The figure shows three views and two pictorial views of one solid part (mm, origin at its lowest corner). Answer the questions. Coordinates: 2 decimals unless noted, no trailing zeros. Loops run counter-clockwise (first coordinate to the right, second up) from the corner with the lowest first, then second, coordinate; pieces in that order, holes last. Notation, with made-up numbers: (55.25, 58) -> (81.25, 58) arc R14 ccw to (81.25, 71) -> close; hole circle Ø8 at (30, 28). An arc over 180 degrees is marked (long way). Answer as a JSON object with one key per item and string values. Group by question number.
1) Section B-B, the plane y = 1.5 is taken. Give the vertices of the cut face in (x, z), plus the area to 3 significant figures.
2) Determine the mould class of the marked faces 1 and 2 for opening direction Z: released by +Z, released by -Z, zero draft, split by the parting line, or undercut.
3) Flat-ended cylindrical pins translate along their axes: P1, Ø6, axis at x = 64.5, y = 3, coming from the +Z side; P2, Ø5, axis at y = 3, z = 43.5, coming from the +X side; P3, Ø1.5, axis at y = 3.5, z = 138.5, coming from the -X side; P4, Ø2, axis at y = 6.5, z = 99, coming from the +X side. Find the tip coordinate at first contact, or state that the pin passes through.
4) Section C-C, the plane x = 118 is taken. Give the vertices of the cut face in (y, z), plus the area to 3 significant figures.
5) Consider probe 1 along Z at (x, y) = (99, 9) (3 decimals); probe 2 along Z at (x, y) = (123, 3.25); probe 3 along Z at (x, y) = (97.5, 1.25). Determine where each line is inside the solid, lowest interval first. Write a range as [from, to].
6) Section A-A, the plane z = 160 is taken. Give the vertices of the cut face in (x, y).
7) Section D-D, the plane z = 100 is taken. Give the vertices of the cut face in (x, y), plus the area to 3 significant figures.
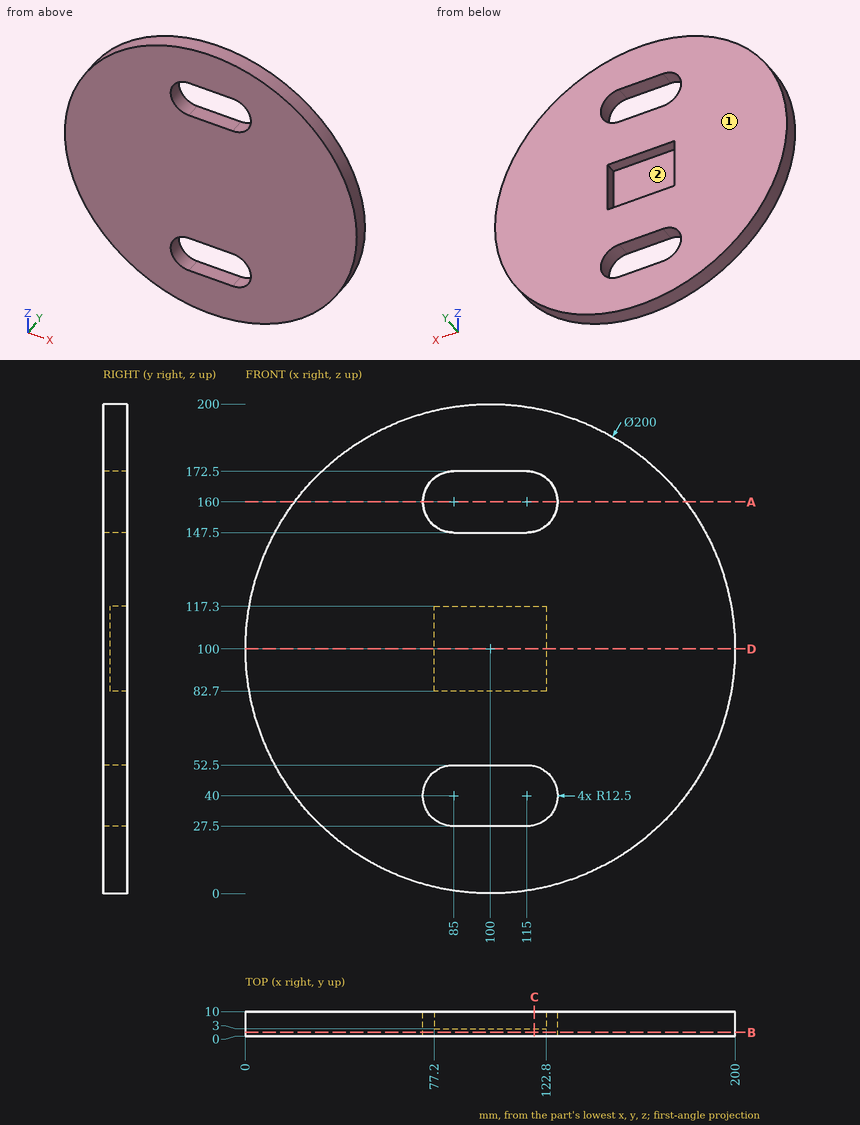
Determined:
{
 "1": {"outline": "circle Ø200 at (100, 100); hole (85, 27.5) -> (115, 27.5) arc R12.5 ccw to (115, 52.5) -> (85, 52.5) arc R12.5 ccw to start; hole (85, 147.5) -> (115, 147.5) arc R12.5 ccw to (115, 172.5) -> (85, 172.5) arc R12.5 ccw to start", "area": "28,900 mm²"},
 "2": {"face 1": "zero draft", "face 2": "undercut"},
 "3": {"P1": "z = 194.57", "P2": "x = 184.17", "P3": "x = 7.4", "P4": "x = 200"},
 "4": {"outline": "(0, 1.63) -> (10, 1.63) -> (10, 27.87) -> (0, 27.87) -> close; (0, 52.13) -> (10, 52.13) -> (10, 82.7) -> (3, 82.7) -> (3, 117.3) -> (10, 117.3) -> (10, 147.87) -> (0, 147.87) -> close; (0, 172.13) -> (10, 172.13) -> (10, 198.37) -> (0, 198.37) -> close", "area": "1,240 mm²"},
 "5": {"probe 1": "[0.005, 27.5], [52.5, 82.7], [117.3, 147.5], [172.5, 199.995]", "probe 2": "[2.68, 30.4], [49.6, 150.4], [169.6, 197.32]", "probe 3": "[0.03, 27.5], [52.5, 147.5], [172.5, 199.97]"},
 "6": {"outline": "(20, 0) -> (72.5, 0) -> (72.5, 10) -> (20, 10) -> close; (127.5, 0) -> (180, 0) -> (180, 10) -> (127.5, 10) -> close"},
 "7": {"outline": "(0, 0) -> (200, 0) -> (200, 10) -> (122.8, 10) -> (122.8, 3) -> (77.2, 3) -> (77.2, 10) -> (0, 10) -> close", "area": "1,680 mm²"}
}
